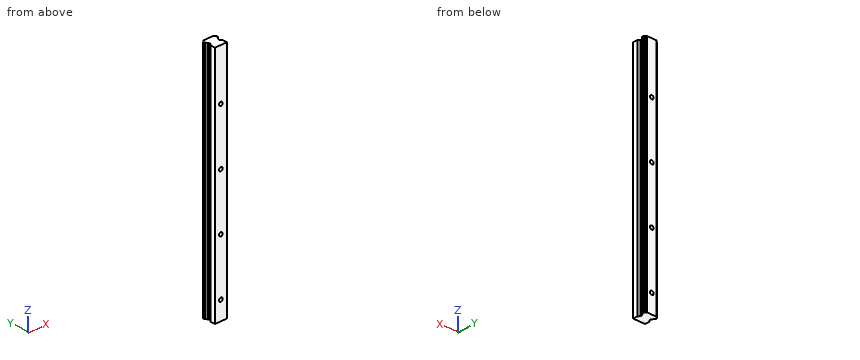
```python
from build123d import *

# Parameters (mm, degrees)
BOSS_EXTRUDE1_DEPTH = 254
SKETCH2_R           = 2
CUT_EXTRUDE1_DEPTH  = 16


with BuildPart() as part:
    # Sketch1 → Boss-Extrude1 (new body)
    with BuildSketch(Plane.XY):
        with BuildLine():
            Line((-6.5, 0), (6.5, 0))
            Line((6.5, 0), (6.5, 5.2))
            Line((6.5, 5.2), (4.8, 6.9))
            Line((4.8, 6.9), (4.8, 8.84))
            Line((4.8, 8.84), (5.754868434, 9.794868434))
            ThreePointArc((5.754868434, 9.794868434), (6.196913421, 10.683086579), (7.085131566, 11.125131566))
            Line((7.085131566, 11.125131566), (7.5, 11.54))
            Line((7.5, 11.54), (7.5, 12.85))
            Line((7.5, 12.85), (7.08164233, 13.26835767))
            ThreePointArc((7.08164233, 13.26835767), (6.196913421, 13.709913421), (5.75535767, 14.59464233))
            Line((5.75535767, 14.59464233), (5.35, 15))
            Line((5.35, 15), (-5.35, 15))
            Line((-5.35, 15), (-5.75535767, 14.59464233))
            ThreePointArc((-5.75535767, 14.59464233), (-6.196913421, 13.709913421), (-7.08164233, 13.26835767))
            Line((-7.08164233, 13.26835767), (-7.5, 12.85))
            Line((-7.5, 12.85), (-7.5, 11.54))
            Line((-7.5, 11.54), (-7.085131566, 11.125131566))
            ThreePointArc((-7.085131566, 11.125131566), (-6.196913421, 10.683086579), (-5.754868434, 9.794868434))
            Line((-5.754868434, 9.794868434), (-4.8, 8.84))
            Line((-4.8, 8.84), (-4.8, 6.9))
            Line((-4.8, 6.9), (-6.5, 5.2))
            Line((-6.5, 5.2), (-6.5, 0))
        make_face()
    extrude(amount=BOSS_EXTRUDE1_DEPTH)

    # Sketch2 → Cut-Extrude1 (cut, through all)
    with BuildSketch(Plane(origin=(0, 15, 0), x_dir=(1, 0, 0), z_dir=(0, 1, 0))):
        with Locations((0, -20)):
            Circle(SKETCH2_R)
        with Locations((0, -79.944)):
            Circle(SKETCH2_R)
        with Locations((0, -139.888)):
            Circle(SKETCH2_R)
        with Locations((0, -199.832)):
            Circle(SKETCH2_R)
    extrude(amount=-CUT_EXTRUDE1_DEPTH, mode=Mode.SUBTRACT)


solid = part.part
```
Could you check a few things on this model? Use its own coordinates, in mm. Round coordinates to 2 decimals unless told otherwise and drop trailing zeros. Loops run counter-clockwise (first coordinate to the right, second up) from the corner with the lowest first, then second, coordinate; pieces in that order, holes last. Notation, with made-up numbers: M -17,-11.75 L -10,-11.75 A27 cw -10,10.25 Z; hole C -27.5,30 d8. An arc over 180 degrees is marked long. Answer as CSV lines item,"result".
1) For pin 1 Ø3.5 at (x, z) = (0, 20) entering from -Y; pin 2 Ø6.5 at (x, z) = (0, 79.944) entering from +Y; pin 3 Ø5.5 at (y, z) = (4, 125.5) entering from +X; pin 4 Ø2.5 at (y, z) = (1.5, 72.5) entering from -X, each with a flat end and sliding along its axis, tell me the tip position at first contact or that it passes through.
From the geometry:
pin 1,"through"
pin 2,"y = 15"
pin 3,"x = 6.5"
pin 4,"x = -6.5"
2) If I drill on probe 1 along Z at (x, y) = (0, 11.5); probe 2 along X at (y, z) = (11.5, 20); probe 3 along Y at (x, z) = (-5.25, 45), over which ranges is the centre line in solid material (lowest first)?
From the geometry:
probe 1,"0 to 18, 22 to 77.94, 81.94 to 137.89, 141.89 to 197.83, 201.83 to 254"
probe 2,"-7.46 to -2, 2 to 7.46"
probe 3,"0 to 6.45, 9.29 to 15"
3) Imagine slicing it at A-A on z = 49. List the corners of the cut face in (x, y) for me, and give its area (3 significant figures).
From the geometry:
outline,"M -7.5,11.54 L -7.09,11.13 A1.56 cw -5.75,9.79 L -4.8,8.84 L -4.8,6.9 L -6.5,5.2 L -6.5,0 L 6.5,0 L 6.5,5.2 L 4.8,6.9 L 4.8,8.84 L 5.75,9.79 A1.56 cw 7.09,11.13 L 7.5,11.54 L 7.5,12.85 L 7.08,13.27 A1.56 cw 5.76,14.59 L 5.35,15 L -5.35,15 L -5.76,14.59 A1.56 cw -7.08,13.27 L -7.5,12.85 Z"
area,"184 mm^2"
